Autodesk Inventor part; units mm, degrees
ref_plane "Plano de trabajo1" through (-77.1004, 28.9483, 0) normal (0, 0, -1) x (-1, 0, 0)
ref_plane "Plano de trabajo3" through (-77.1004, 28.9483, 0) normal (0, 0, 1) x (1, 0, 0)
ref_plane "Plano de trabajo2" through (-77.1004, 28.9483, -20) normal (0, 0, -1) x (-1, 0, 0)
ref_plane "Plano de trabajo1" through (-77.1004, 28.9483, 0) normal (0, 0, -1) x (-1, 0, 0)
sketch "Boceto1" plane through (-77.1004, 28.9483, 0) normal (0, 0, -1) x (-1, 0, 0)
  line L0 (82, -56) -> (-3, -56)
  line L1 (-3, -56) -> (-3, 0)
  line L2 (-3, 0) -> (82, 0)
  line L3 (82, 0) -> (82, -56)
  point P0 (-77.1004, -28.9483)
extrude "Extrusión1" add sketch "Boceto1" along normal blind 20
ref_plane "Plano de trabajo3" through (-77.1004, 28.9483, 0) normal (0, 0, 1) x (1, 0, 0)
sketch "Boceto2" plane through (-77.1004, 28.9483, 0) normal (0, 0, 1) x (1, 0, 0)
  circle A0 centre (-78.5, -3.5) radius 1.375
  circle A1 centre (-78.5, -3.5) radius 1.125
  circle A2 centre (-20.5, -3.5) radius 1.375
  circle A3 centre (-20.5, -3.5) radius 1.125
  circle A4 centre (-20.5, -52.5) radius 1.375
  circle A5 centre (-20.5, -52.5) radius 1.125
  circle A6 centre (-78.5, -52.5) radius 1.375
  circle A7 centre (-78.5, -52.5) radius 1.125
  line L0 (-91.1268, 5.8368) -> (25.5851, 5.8368)
  line L1 (25.5851, 5.8368) -> (25.5851, -70.6743)
  line L2 (25.5851, -70.6743) -> (-91.1268, -70.6743)
  line L3 (-91.1268, -70.6743) -> (-91.1268, 5.8368)
  point P0 (77.1004, -28.9483)
  dimension "d3" = 2.25
  dimension "d4" = 2.25
  dimension "d5" = 2.25
  dimension "d6" = 2.25
extrude "Extrusión2" cut sketch "Boceto2" against normal blind 10 contours L0 L1 L2 L3
ref_plane "Plano de trabajo2" through (-77.1004, 28.9483, -20) normal (0, 0, -1) x (-1, 0, 0)
sketch "Boceto8" plane through (-77.1004, 28.9483, -20) normal (0, 0, -1) x (-1, 0, 0)
  circle A0 centre (77, -33) radius 1.25
  circle A1 centre (77, -5) radius 1.25
  line L0 (-3, -56) -> (82, -56)
  circle A2 centre (5, -33) radius 1.25
  circle A3 centre (5, -5) radius 1.25
  line L1 (82, -56) -> (82, 0)
  line L2 (82, -56) -> (72, -56)
  line L3 (72, -56) -> (72, 0)
  line L4 (72, 0) -> (82, 0)
  line L5 (82, 0) -> (82, -56)
  line L6 (10.1328, -56) -> (0.1328, -56)
  line L7 (5, -33) -> (5, -5)
  line L8 (0, -59.0097) -> (0, -32.6767)
  line L9 (79, -56) -> (0, -56)
  line L10 (0, -56) -> (10, -56)
  line L11 (10, -56) -> (10, 0)
  line L12 (10, 0) -> (0, 0)
  line L13 (0, 0) -> (0, -56)
  line L14 (82, 0) -> (-3, 0)
  point P0 (-77.1004, -28.9483)
  dimension "d31" = 2.5
  dimension "d32" = 2.5
  dimension "d33" = 28
  dimension "d35" = 2.5
  dimension "d36" = 72
  dimension "d37" = 2.5
  dimension "d38" = 5
  dimension "d39" = 72
  dimension "d40" = 5
  dimension "d41" = 28
  dimension "d43" = 10
  dimension "d45" = 5
  dimension "d46" = 10
  dimension "d92" = 0
extrude "Extrusión8" add sketch "Boceto8" along normal blind 30 contours L8 L13 L12 L11 L0 | L3 L4 L1 L0
ref_plane "Plano de trabajo6" through (-159.1004, -27.0517, -10) normal (-1, 0, 0) x (0, 0, 1)
sketch "Boceto9" plane through (-159.1004, -27.0517, -10) normal (-1, 0, 0) x (0, 0, 1)
  line L0 (-29, 31) -> (-40, 31)
  line L1 (-40, 31) -> (-40, 43)
  line L2 (-40, 43) -> (-29, 43)
  line L3 (-29, 43) -> (-29, 31)
  line L4 (0, 0) -> (-40, 0)
  line L5 (-40, 0) -> (-40, 56)
  line L6 (0, 56) -> (-40, 56)
  point P0 (10, 27.0517)
  dimension "d49" = 11
  dimension "d50" = 12
  dimension "d52" = 0
  dimension "d82" = 13
extrude "Extrusión9" cut sketch "Boceto9" against normal blind 100
ref_plane "Plano de trabajo5" through (-149.1004, -27.0517, -20) normal (1, 0, 0) x (0, 0, -1)
sketch "Boceto10" plane through (-149.1004, -27.0517, -20) normal (1, 0, 0) x (0, 0, -1)
  line L0 (17, 29) -> (30, 29)
  line L1 (30, 29) -> (30, 45)
  line L2 (30, 45) -> (17, 45)
  line L3 (17, 45) -> (17, 29)
  line L4 (-10, 56) -> (30, 56)
  line L5 (30, 31) -> (30, 0)
  line L6 (19, 31) -> (19, 43)
  line L7 (30, 31) -> (19, 31)
  line L8 (19, 31) -> (19, 43)
  line L9 (19, 43) -> (30, 43)
  line L10 (19, 43) -> (30, 43)
  point P0 (-20, 27.0517)
  dimension "d59" = 13
  dimension "d60" = 16
extrude "Extrusión10" add sketch "Boceto10" along normal blind 6 contours L3 L2 L1 L9 L6 L7 L0
sketch "Boceto11" plane through (-77.1004, -27.0517, -20) normal (1, 0, 0) x (0, 0, -1)
  line L0 (30, 43) -> (30, 74)
  line L1 (17, 29) -> (30, 29)
  line L2 (30, 29) -> (30, 45)
  line L3 (30, 45) -> (17, 45)
  line L4 (17, 45) -> (17, 29)
  line L5 (30, 31) -> (19, 31)
  line L6 (19, 31) -> (30, 31)
  line L7 (30, 31) -> (19, 31)
  line L8 (19, 31) -> (19, 43)
  line L9 (19, 31) -> (19, 43)
  line L10 (30, 43) -> (19, 43)
  line L11 (19, 43) -> (30, 43)
  line L12 (19, 43) -> (30, 43)
  point P0 (-20, 27.0517)
  point P1 (-20, 27.0517)
  dimension "d64" = 13
  dimension "d65" = 16
  dimension "d66" = 2
  dimension "d88" = 0
  dimension "d89" = 2
extrude "Extrusión11" add sketch "Boceto11" against normal blind 16 contours L10 L8 L5 L2 L1 L4 L3 L0
ref_plane "Plano de trabajo4" through (-159.1004, -27.0517, -10) normal (0, -1, 0) x (1, 0, 0)
sketch "Boceto12" plane through (-159.1004, -27.0517, -10) normal (0, -1, 0) x (1, 0, 0)
  line L0 (0, 0) -> (0, -40)
  line L1 (0, -7) -> (97.2238, -7)
  line L2 (97.2238, -7) -> (97.2238, 2.4478)
  line L3 (97.2238, 2.4478) -> (0, 2.4478)
  line L4 (0, 2.4478) -> (0, -7)
  line L5 (72, -10) -> (10, -10)
  point P0 (159.1004, 10)
  dimension "d69" = 3
extrude "Extrusión12" cut sketch "Boceto12" against normal blind 60
sketch "Boceto13" plane through (-155.6004, 25.4483, 0) normal (0, 0, 1) x (1, 0, 0)
  line L0 (90.0679, 13.1573) -> (-12.4886, 13.1573)
  line L1 (-12.4886, 13.1573) -> (-12.4886, -64.4116)
  line L2 (-12.4886, -64.4116) -> (90.0679, -64.4116)
  line L3 (90.0679, -64.4116) -> (90.0679, 13.1573)
  point P0 (155.6004, -25.4483)
extrude "Extrusión13" cut sketch "Boceto13" against normal blind 10
ref_plane "Plano de trabajo8" through (-159.1004, -27.0517, -17) normal (0, 0, 1) x (1, 0, 0)
sketch "Boceto14" plane through (-159.1004, -27.0517, -17) normal (0, 0, 1) x (1, 0, 0)
  circle A0 centre (61.5, 52.5) radius 1.375
  circle A1 centre (61.5, 52.5) radius 1.375
  circle A2 centre (61.5, 3.5) radius 1.375
  circle A3 centre (61.5, 3.5) radius 1.375
  circle A4 centre (3.5, 3.5) radius 1.375
  circle A5 centre (3.5, 3.5) radius 1.375
  circle A6 centre (3.5, 52.5) radius 1.375
  circle A7 centre (3.5, 52.5) radius 1.375
  point P0 (159.1004, 27.0517)
extrude "Extrusión14" cut sketch "Boceto14" against normal blind 10
ref_plane "Plano de trabajo7" through (-159.1004, -27.0517, -17) normal (0, 0, 1) x (1, 0, 0)
sketch "Boceto15" plane through (-159.1004, -27.0517, -17) normal (0, 0, 1) x (1, 0, 0)
  circle A0 centre (61.5, 52.5) radius 1.375
  circle A1 centre (61.5, 52.5) radius 2.5
  circle A2 centre (61.5, 3.5) radius 1.375
  circle A3 centre (61.5, 3.5) radius 2.5
  circle A4 centre (3.5, 3.5) radius 1.375
  circle A5 centre (3.5, 3.5) radius 2.5
  circle A6 centre (3.5, 52.5) radius 1.375
  circle A7 centre (3.5, 52.5) radius 2.5
  point P0 (159.1004, 27.0517)
  dimension "d76" = 5
  dimension "d77" = 5
  dimension "d78" = 5
  dimension "d79" = 5
extrude "Extrusión15" add sketch "Boceto15" along normal blind 3
sketch "Boceto16" plane through (-149.1004, -27.0517, -20) normal (0, -1, 0) x (1, 0, 0)
  line L0 (-10, 3) -> (-10, -30)
  line L1 (-10, 3) -> (-37, 3)
  line L2 (-37, 3) -> (-37, 0)
  line L3 (-37, 0) -> (-10, 0)
  line L4 (-10, 0) -> (-10, 3)
  point P0 (149.1004, 20)
  dimension "d93" = 27
  dimension "d94" = 3
extrude "Extrusión16" add sketch "Boceto16" against normal blind 67
sketch "Boceto17" plane through (-74.1004, -27.0517, -17) normal (0, 0, 1) x (1, 0, 0)
  line L0 (-85.9191, 67.0002) -> (-111.9991, 67.0002)
  line L1 (-111.9991, 67.0002) -> (-111.9991, 5.5802)
  line L2 (-111.9991, 5.5802) -> (-85.9191, 5.5802)
  line L3 (-85.9191, 5.5802) -> (-85.9191, 67.0002)
  line L4 (-91.7766, 36.2902) -> (-98.9591, 36.2902)
  line L5 (-98.9591, 36.2902) -> (-98.9591, 28.1123)
  circle A0 centre (-88.4591, 64.5402) radius 1.25
  circle A1 centre (-88.4591, 8.0402) radius 1.25
  circle A2 centre (-109.4591, 64.5402) radius 1.25
  circle A3 centre (-109.4591, 8.0402) radius 1.25
  point P0 (74.1004, 27.0517)
  dimension "d97" = 26.08
  dimension "d98" = 61.42
  dimension "d99" = 2.5
  dimension "d100" = 28.25
  dimension "d101" = 10.5
extrude "Extrusión17" cut sketch "Boceto17" against normal blind 56 contours A0 | A1 | A2 | A3
sketch "Boceto18" plane through (-74.1004, -27.0517, -17) normal (0, 0, 1) x (1, 0, 0)
  circle A0 centre (-109.4591, 64.5402) radius 1.25
  circle A1 centre (-88.4591, 64.5402) radius 1.25
  circle A2 centre (-88.4591, 8.0402) radius 1.25
  circle A3 centre (-109.4591, 8.0402) radius 1.25
  circle A4 centre (-81.5, 3.5) radius 2.5
  circle A5 centre (-23.5, 52.5) radius 2.5
  circle A6 centre (-23.5, 3.5) radius 2.5
  circle A7 centre (-81.5, 52.5) radius 2.5
  line L0 (0, 56) -> (0, 0)
  line L1 (-85, 56) -> (0, 56)
  line L2 (-85, 56) -> (-85, 67)
  line L3 (-112, 67) -> (-85, 67)
  line L4 (-112, 0) -> (-112, 67)
  line L5 (0, 0) -> (-112, 0)
  circle A8 centre (-88.4591, 64.5402) radius 2.25
  circle A9 centre (-109.4591, 64.5402) radius 2.25
  circle A10 centre (-88.4591, 8.0402) radius 2.25
  circle A11 centre (-109.4591, 8.0402) radius 2.25
  point P0 (74.1004, 27.0517)
  dimension "d104" = 5
  dimension "d105" = 4.5
  dimension "d106" = 4.5
  dimension "d107" = 4.5
  dimension "d108" = 4.5
extrude "Extrusión18" add sketch "Boceto18" along normal blind 3 contours A8 | A9 | A10 | A11
fillet "Empalme1" radius 4 1 edges at (-186.1004, -27.0517, -18.5)
sketch "Boceto19" plane through (-74.1004, -27.0517, -17) normal (0, 0, 1) x (1, 0, 0)
  line L0 (-85, 0) -> (-85, 31)
  line L1 (-85, 4.711) -> (-113.131, 4.711)
  line L2 (-113.131, 4.711) -> (-113.131, -0.5367)
  line L3 (-113.131, -0.5367) -> (-85, -0.5367)
  line L4 (-85, -0.5367) -> (-85, 4.711)
  point P0 (74.1004, 27.0517)
extrude "Extrusión19" cut sketch "Boceto19" against normal blind 3
fillet "Empalme2" radius 4 1 edges at (-186.1004, -22.3407, -18.5)
fillet "Empalme3" radius 3 2 edges at (-159.1004, 39.9483, -18.5) (-186.1004, 39.9483, -18.5)
properties part number "baseRaspberry"
Source: CAD feature listing. Evaluate the final solid. Frame: model axes, mm. A direction names the side the tool comes from. Give positions to 0.01 mm unless a question says otherwise; leave off trailing zeros. Write each loop counter-clockwise with the first axis right and the second up, starting at its lowest first coordinate (ties: lowest second). Pieces come first, ordered by that corner, then holes. Notation, with made-up numbers: M 59,70 L 115,70 A28 ccw 115,101 Z; hole C -32,64.5 d9. An arc over 180 degrees is marked long. Return JSON: item names as keys, results as strings. Group by question number.
1) Cut plane A-A, the plane z = -35. Output: boundary loops of the cut face in (x, y), plus the area to 3 significant figures.
2) Cut plane D-D, the plane z = -25.5. Output: boundary loops of the cut face in (x, y) (3 decimals), plus the area to 3 significant figures.
3) Set-up query: faces 5 (the face through (-120, 28.948, -19)), 6 (the face through (-77.1, 1, -35)), 7 (the face through (-185.807, -19.11, -15.521)), 8 (the face through (-146, 1.948, -43)). Return all of +Z, -Z, +X, -X, +Y, -Y with unobstructed straight access to the full face (end or side cutting, diameter ignored); none if empty.
4) Cut plane B-B, the plane y = -7. Output: boundary loops of the cut face in (x, z), plus the area to 3 significant figures.
5) Pull-direction query (Y, two-part tool) for faces 1 (the face through (-152.85, -4.11, -34.79)), 2 (the face through (-184.9, -21.2, -18.5)), 3 (the face through (-81.83, 25.17, -34.79)), 4 (the face through (-184, 36, -14)); classes: pulls with the +Y half, pulls with the -Y half, needs draft (parallel to the pull), parting line crosses it, or undercut.
6) Pin query (flat end, axial travel): P1, Ø1.2, axis at x = -82, y = -4, coming from the -Z side; P2, Ø3, axis at x = -90, y = 8, coming from the +Z side; P3, Ø5, axis at x = -142, z = -24.5, coming from the -Y side; P4, Ø1.8, axis at x = -144.5, z = -42, coming from the -Y side. Return the tip coordinate at first contact, or that it passes through.
7) Material intervals for line 1 along X through (y, z) = (-20, -35); line 2 along X through (y, z) = (25, -33.5); line 3 along X through (y, z) = (24.5, -23.5), sorted ascending. Write a range as [from, to].
8) Cut plane C-C, the plane z = -40.5. Output: boundary loops of the cut face in (x, y).
Recorded:
{
 "1": {"outline": "M -159.1,-27.05 L -149.1,-27.05 L -149.1,28.95 L -159.1,28.95 Z; M -87.1,-27.05 L -77.1,-27.05 L -77.1,28.95 L -87.1,28.95 Z; hole C -154.1,-4.05 d2.5; hole C -154.1,23.95 d2.5; hole C -82.1,-4.05 d2.5; hole C -82.1,23.95 d2.5", "area": "1,100 mm²"},
 "2": {"outline": "M -159.1,-27.052 L -149.1,-27.052 L -149.1,28.948 L -159.1,28.948 Z; M -87.1,-27.052 L -77.1,-27.052 L -77.1,28.948 L -87.1,28.948 Z; hole C -155.6,-23.552 d2.75; hole C -154.1,-4.052 d2.5; hole M -155.341,24.098 A1.25 ccw long -154.25,25.189 A1.375 ccw long Z; hole C -82.1,-4.052 d2.5; hole C -82.1,23.948 d2.5", "area": "1,090 mm²"},
 "3": {"face 5": "+Z, -Z, +X, +Y", "face 6": "-Z, +X, +Y, -Y", "face 7": "+Z", "face 8": "-Z, -Y"},
 "4": {"outline": "M -186.1,-20 L -159.1,-20 L -159.1,-50 L -149.1,-50 L -149.1,-20 L -87.1,-20 L -87.1,-50 L -77.1,-50 L -77.1,-20 L -74.1,-20 L -74.1,-17 L -186.1,-17 Z", "area": "936 mm²"},
 "5": {"face 1": "undercut", "face 2": "pulls with the -Y half", "face 3": "undercut", "face 4": "needs draft"},
 "6": {"P1": "stops at z = -20", "P2": "stops at z = -17", "P3": "passes through", "P4": "stops at y = 1.95"},
 "7": {"line 1": "x = [-159.1, -149.1], [-87.1, -77.1]", "line 2": "x = [-159.1, -154.78], [-153.42, -149.1], [-87.1, -82.78], [-81.42, -77.1]", "line 3": "x = [-159.1, -156.6], [-152.98, -149.1], [-87.1, -83.22], [-80.98, -77.1]"},
 "8": {"outline": "M -159.1,-27.05 L -149.1,-27.05 L -149.1,1.95 L -143.1,1.95 L -143.1,3.95 L -159.1,3.95 Z; M -159.1,15.95 L -143.1,15.95 L -143.1,17.95 L -149.1,17.95 L -149.1,28.95 L -159.1,28.95 Z; M -93.1,1.95 L -87.1,1.95 L -87.1,-27.05 L -77.1,-27.05 L -77.1,3.95 L -93.1,3.95 Z; M -93.1,15.95 L -77.1,15.95 L -77.1,28.95 L -87.1,28.95 L -87.1,17.95 L -93.1,17.95 Z; hole C -154.1,-4.05 d2.5; hole C -154.1,23.95 d2.5; hole C -82.1,-4.05 d2.5; hole C -82.1,23.95 d2.5"}
}
